For this review, take the finished solid that the model builds, in its own axes (mm). A direction names the side the tool comes from. Coordinates: 2 decimals unless noted, no trailing zeros. Order: outer loops, then holes, each group sorted by start corner. A loop starts at its lowest first (then second) coordinate and runs counter-clockwise, first axis right, second up. Notation, with made-up numbers: M 6,-4.5 L 10,-4.5 A12 cw 10,3.5 Z; hole C 12,-39 d5. An arc over 180 degrees is marked long. Use CSV: the item, a comma, the result in double quotes.
Autodesk Inventor part; units mm, degrees
ref_plane "YZ Plane" through (0, 0, 0) normal (1, 0, 0) x (0, 1, 0)
ref_plane "XZ Plane" through (0, 0, 0) normal (0, 1, 0) x (-1, 0, 0)
ref_plane "XY Plane" through (0, 0, 0) normal (0, 0, 1) x (1, 0, 0)
sketch "Sketch1" plane through (0, 0, 0) normal (0, 1, 0) x (-1, 0, 0)
  line L0 (0, 0) -> (-36, 0)
  line L1 (-36, -14) -> (0, -14)
  line L2 (0, 0) -> (0, -2.5)
  line L3 (-2, -2.5) -> (-2, -11.5)
  line L4 (-34, -2.5) -> (-34, -11.5)
  line L5 (0.1666, -2.5) -> (-2, -2.5)
  line L6 (0, -14) -> (0, -11.5)
  line L7 (0, -11.5) -> (-2, -11.5)
  line L8 (-34, -11.5) -> (-36, -11.5)
  line L9 (-36, -11.5) -> (-36, -14)
  line L10 (-34, -2.5) -> (-36, -2.5)
  line L11 (-36, -2.5) -> (-36, 0)
  dimension "d1" = 14
  dimension "d2" = 36
  dimension "d3" = 2.5
  dimension "d4" = 9
  dimension "d5" = 9
  dimension "d6" = 32
  dimension "d8" = 9
  dimension "d9" = 36
extrude "Extrusion1" add sketch "Sketch1" along normal blind 36
sketch "Sketch2" plane through (0, 36, 0) normal (0, 1, 0) x (1, 0, 0)
  circle A0 centre (18, 7) radius 1.25
  line L0 (34, 2.5) -> (34, 11.5)
  line L1 (0, 0) -> (36, 0)
  dimension "d12" = 2.5
  dimension "d13" = 16
  dimension "d14" = 7
sketch "Sketch3" plane through (0, 0, 0) normal (0, 0, 1) x (1, 0, 0)
  circle A0 centre (18, 18) radius 11
  circle A1 centre (18, 18) radius 9
  line L0 (0, 0) -> (36, 0)
  line L1 (0, 0) -> (0, 36)
  dimension "d15" = 22
  dimension "d16" = 18
  dimension "d17" = 18
  dimension "d18" = 18
hole "Hole1" at (18, 18, 0) direction (0, 0, -1) diameter 18 end through all
extrude "Extrusion2" add sketch "Sketch3" along normal blind 0.2
hole "Hole2" at (18, 36, -7) direction (0, -1, 0) diameter 2.5 end up to surface countersink diameter 4 countersink angle 90
properties part number "HUDSON 1-08 AXLE BLOCK"
Item 1: Clearance check with flat-ended pins moving along their axes: pin 1 Ø2.5 at (y, z) = (11, -9) entering from -X; pin 2 Ø11 at (x, y) = (18, 18) entering from +Z; pin 3 Ø0.6 at (x, y) = (1, 21.5) entering from +Z; pin 4 Ø2 at (x, z) = (18, -7) entering from +Y. State where each tip first meets the part, or that it passes through.
Solutions:
pin 1,"x = 2"
pin 2,"through"
pin 3,"z = 0"
pin 4,"y = 9.06"
Item 2: For faces 4 (the face through (1, 18, -11.5)), 5 (the face through (22.3, 9.7, -14)), 6 (the face through (10, 10, 0)), 7 (the face through (35, 18, -11.5)), list the 3-axis set-ups (+Z, -Z, +X, -X, +Y, -Y) from which the entire face can be reached by the end or side of a thin tool; tool diameter is ignored.
Solutions:
face 4,"-X, +Y, -Y"
face 5,"-Z, +X, -X, +Y, -Y"
face 6,"+Z"
face 7,"+X, +Y, -Y"
Item 3: Add section A-A on z = -12.5. State the section outline as (x, y) points.
Solutions:
outline,"M 0,0 L 36,0 L 36,36 L 0,36 Z; hole C 18,18 d18"
Item 4: Add section C-C on z = -7. State the section outline as (x, y) points, and give its area (3 significant figures).
Solutions:
outline,"M 2,0 L 34,0 L 34,36 L 20,36 L 19.25,35.25 L 19.25,26.91 A9 cw long 16.75,26.91 L 16.75,35.25 L 16,36 L 2,36 Z"
area,"874 mm^2"
Item 5: To check wall thickness, follow line 1 along X through (y, z) = (18, -7.75); line 2 along Z through (x, y) = (3, 7); line 3 along X through (y, z) = (6.5, -9.25). State the ranges of each line that lie inside material, in increasing order. Write a range as [from, to].
Solutions:
line 1,"[2, 9], [27, 34]"
line 2,"[-14, 0]"
line 3,"[2, 34]"
Item 6: Add section B-B on y = 32.5. State the section outline as (x, z) points.
Solutions:
outline,"M 0,-14 L 36,-14 L 36,-11.5 L 34,-11.5 L 34,-2.5 L 36,-2.5 L 36,0 L 0,0 L 0,-2.5 L 2,-2.5 L 2,-11.5 L 0,-11.5 Z; hole C 18,-7 d2.5"
Item 7: Draft analysis for pull direction X (two halves, no side actions). For faces 1 (the face through (36, 18, -1)), 2 (the face through (17.155, 31.023, -7.921)), 3 (the face through (18, 0, -7)), state which applies: released by +X, released by -X, zero draft, split by the parting line, or undercut.
Solutions:
face 1,"released by +X"
face 2,"undercut"
face 3,"zero draft"
Item 8: Add section D-D on y = 5. State the section outline as (x, z) points.
Solutions:
outline,"M 0,-14 L 36,-14 L 36,-11.5 L 34,-11.5 L 34,-2.5 L 36,-2.5 L 36,0 L 0,0 L 0,-2.5 L 2,-2.5 L 2,-11.5 L 0,-11.5 Z"
